Drawing for the job (mm, zero at the part's lowest x, y, z). A direction names the side the tool comes from. Coordinates: 2 decimals unless noted, no trailing zeros. Write each loop counter-clockwise with the first axis right and the second up, starting at its lowest first coordinate (ties: lowest second). Pieces come first, ordered by that corner, then holes. Notation, with made-up numbers: (81, 14) -> (104, 14) arc R11 cw to (104, 23) -> close; hole circle Ø1 at (83, -0.75). An arc over 180 degrees is marked (long way). Answer as CSV lines item,"result".
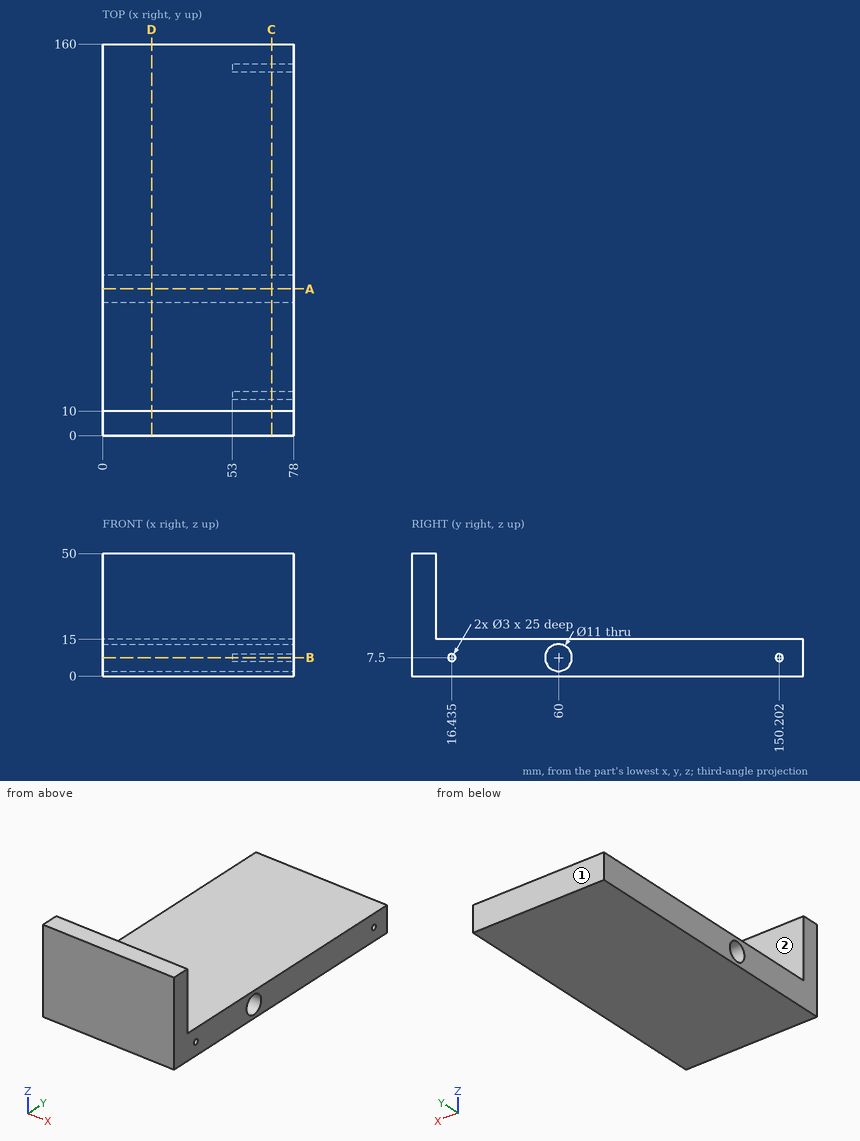
Item 1: Saw through at B-B on z = 7.5. Give the cut face in (x, y) (1 decimal).
Answer below:
outline,"(0, 0) -> (78, 0) -> (78, 14.9) -> (53, 14.9) -> (53, 17.9) -> (78, 17.9) -> (78, 54.5) -> (0, 54.5) -> close; (0, 65.5) -> (78, 65.5) -> (78, 148.7) -> (53, 148.7) -> (53, 151.7) -> (78, 151.7) -> (78, 160) -> (0, 160) -> close"
Item 2: Saw through at C-C on x = 69. Give the cut face in (y, z) (1 decimal), and give its area (3 significant figures).
Answer below:
outline,"(0, 0) -> (160, 0) -> (160, 15) -> (10, 15) -> (10, 50) -> (0, 50) -> close; hole circle Ø3 at (16.4, 7.5); hole circle Ø11 at (60, 7.5); hole circle Ø3 at (150.2, 7.5)"
area,"2,640 mm2"
Item 3: Flat gauge pins, fed straight in: pin 1 (1 mm diameter, centred on x = 23.5, z = 39, fed in from +Y); pin 2 (1.5 mm diameter, centred on y = 16, z = 7, fed in from +X); pin 3 (1.5 mm diameter, centred on x = 66.5, y = 93, fed in from +Z). Where does each tip first touch, or does it go through?
Answer below:
pin 1,"stops at y = 10"
pin 2,"stops at x = 53"
pin 3,"stops at z = 15"
Item 4: Saw through at A-A on y = 60. Give the cut face in (x, z), and give its area (3 significant figures).
Answer below:
outline,"(0, 0) -> (78, 0) -> (78, 2) -> (0, 2) -> close; (0, 13) -> (78, 13) -> (78, 15) -> (0, 15) -> close"
area,"312 mm2"
Item 5: Wall check: line 1 (Z direction, x = 54.5, y = 60); line 2 (Y direction, x = 30, z = 7); line 3 (Z direction, x = 4.5, y = 121). Give the ranges that are in metal, low to high. Write a range as from..to.
Answer below:
line 1,"z = 0..2, 13..15"
line 2,"y = 0..54.52, 65.48..160"
line 3,"z = 0..15"
Item 6: 3-axis set-ups, long thin cutter, end or side, ignore diameter. For the marked faces 1 and 2: which of +Z, -Z, +X, -X, +Y, -Y reach the whole face in a straight line?
Answer below:
face 1,"+Z, -Z, +X, -X, +Y"
face 2,"+Z, +X, -X, +Y"
Item 7: Saw through at D-D on x = 20. Give the cut face in (y, z), and give its area (4 significant figures).
Answer below:
outline,"(0, 0) -> (160, 0) -> (160, 15) -> (10, 15) -> (10, 50) -> (0, 50) -> close; hole circle Ø11 at (60, 7.5)"
area,"2,655 mm2"
